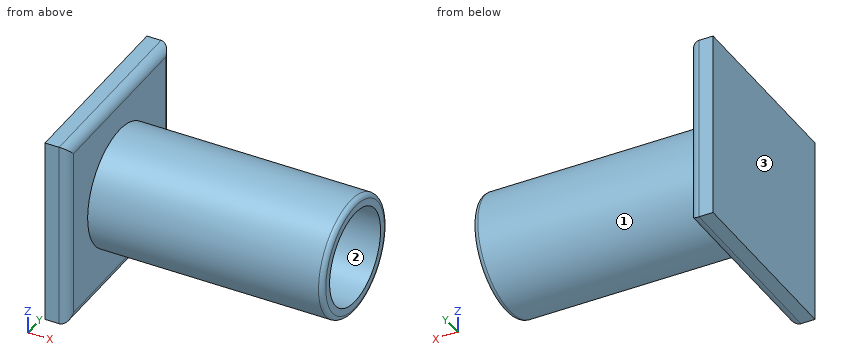
```python
from build123d import *

# Parameters (mm, degrees)
SKETCH3_W           = 800
SKETCH3_H           = 800
BOSS_EXTRUDE1_DEPTH = 100
SKETCH4_R           = 250
SKETCH4_R_2         = 200
BOSS_EXTRUDE2_DEPTH = 1000
FILLET3_R           = 40
FILLET4_R           = 20


with BuildPart() as part:
    # Sketch3 → Boss-Extrude1 (new body)
    with BuildSketch(Plane(origin=(0, 0, 0), x_dir=(0, 0, -1), z_dir=(1, 0, 0))):
        Rectangle(SKETCH3_W, SKETCH3_H)
    extrude(amount=BOSS_EXTRUDE1_DEPTH)

    # Sketch4 → Boss-Extrude2 (add)
    with BuildSketch(Plane(origin=(100, 0, 0), x_dir=(0, 0, -1), z_dir=(1, 0, 0))):
        with Locations(Location((0, 0, 0), (0, 0, 180))):
            Circle(SKETCH4_R)
        Circle(SKETCH4_R_2, mode=Mode.SUBTRACT)
    extrude(amount=BOSS_EXTRUDE2_DEPTH)

    # Fillet3
    fillet3_edges = [part.edges().sort_by_distance(p)[0] for p in [
        (100, 0, 400),
        (100, -400, 0),
        (100, 0, -400),
        (100, 400, 0),
    ]]
    fillet(fillet3_edges, radius=FILLET3_R)

    # Fillet4
    fillet4_edges = [part.edges().sort_by_distance(p)[0] for p in [
        (1100, 0, -250),
    ]]
    fillet(fillet4_edges, radius=FILLET4_R)


solid = part.part
```
The model under review builds one solid part; all positions refer to its coordinate system, in mm. Face numbers are marked on the shaded views. Give positions to 0.01 mm unless a question says otherwise; leave off trailing zeros. Write each loop counter-clockwise with the first axis right and the second up, starting at its lowest first coordinate (ties: lowest second). Pieces come first, ordered by that corner, then holes. Notation, with made-up numbers: (66.5, -13) -> (95.5, -13) arc R31 cw to (95.5, 15) -> close; hole circle Ø10 at (3, 16.25). An arc over 180 degrees is marked (long way). Put each result on its own line as item: value.
(1) We need section C-C, the plane x = 703.5. Give the boundary of the cut face in (y, z).
Results are:
outline: circle Ø500 at (0, 0); hole circle Ø400 at (0, 0)
(2) To check wall thickness, follow probe 1 along Y at (x, z) = (775, 0); probe 2 along Z at (x, y) = (903.5, 11); probe 3 along Z at (x, y) = (833, -1.5). State the ranges of each line that lie inside material, in increasing order. Write a range as from..to.
Results are:
probe 1: -250..-200, 200..250
probe 2: -249.76..-199.7, 199.7..249.76
probe 3: -250..-199.99, 199.99..250
(3) The part is to be moulded in two halves that separate along Y. For the marked faces 1, 2 and 3, say which applies: pulls with the +Y half, pulls with the -Y half, needs draft (parallel to the pull), parting line crosses it, or undercut.
Results are:
face 1: parting line crosses it
face 2: undercut
face 3: needs draft
(4) For pin 1 Ø4 at (x, z) = (132, -162.5) entering from +Y; pin 2 Ø4 at (x, y) = (694.5, 58.5) entering from -Z; pin 3 Ø3 at (x, y) = (626.5, -111) entering from +Z, all flat-tipped, find the tip position at first contact; note any pin that passes through.
Results are:
pin 1: y = 191.68
pin 2: z = -243.53
pin 3: z = 224.74
(5) We need section A-A, the plane z = 0. Give the boundary of the cut face in (x, y), and give its area (3 significant figures).
Results are:
outline: (0, -400) -> (60, -400) arc R40 ccw to (100, -360) -> (100, -250) -> (1080, -250) arc R20 ccw to (1100, -230) -> (1100, -200) -> (100, -200) -> (100, 200) -> (1100, 200) -> (1100, 230) arc R20 ccw to (1080, 250) -> (100, 250) -> (100, 360) arc R40 ccw to (60, 400) -> (0, 400) -> close
area: 179,000 mm²
